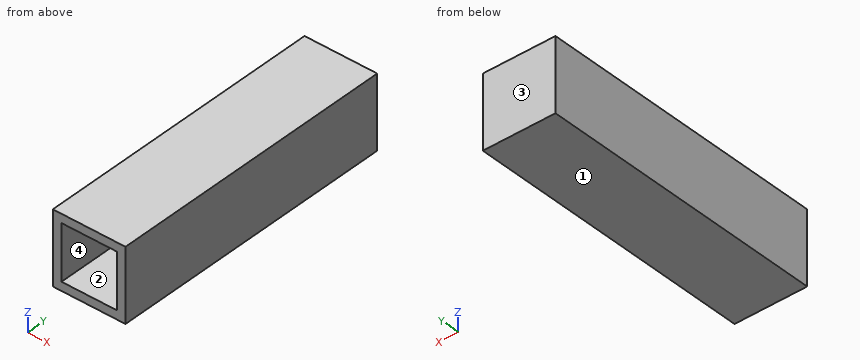
```python
from build123d import *

# Parameters (mm, degrees)
SKETCH2_W             = 25
SKETCH2_H             = 25
BOSS_EXTRUDE2_DEPTH   = 100
SHELL2_T              = -3
BODY_MOVE_COPY1_ANGLE = 180


with BuildPart() as part:
    # Sketch2 → Boss-Extrude2 (new body)
    with BuildSketch(Plane(origin=(0, 0, 0), x_dir=(1, 0, 0), z_dir=(0, 1, 0))):
        Rectangle(SKETCH2_W, SKETCH2_H)
    extrude(amount=BOSS_EXTRUDE2_DEPTH)

    # Shell2
    shell2_openings = [part.faces().sort_by_distance(p)[0] for p in [
        (0, 100, 0),
    ]]
    offset(amount=SHELL2_T, openings=shell2_openings, kind=Kind.INTERSECTION)


with BuildPart() as part_1:
    # Body-Move/Copy1: moved
    add(part.part.rotate(Axis((0, 50, 0), (0, 0, 1)), BODY_MOVE_COPY1_ANGLE))


solid = part_1.part
```
Read the model definition and answer for the solid it produces. Units are mm, in the model's axes. Face numbers are marked on the shaded views. Give positions to 0.01 mm unless a question says otherwise; leave off trailing zeros. Loops run counter-clockwise (first coordinate to the right, second up) from the corner with the lowest first, then second, coordinate; pieces in that order, holes last.
Item 1: This flat-tipped pin is pushed along its axis until it touches: pin 1 Ø1.5 at (x, z) = (-4.5, -1.5) entering from -Y. Where does it stop, or does it pass through?
Item 2: The part is cut by section C-C (z = -8). Write down the section's boundary in (x, y), and give its area (3 significant figures).
Item 3: The part is cut by section B-B (x = -4.5). Write down the section's boundary in (y, z), and give its area (3 significant figures).
Item 4: Find the intervals of material crossed by line 1 along X through (y, z) = (15, 6.75); line 2 along Y through (x, z) = (0.25, -5.5), in increasing order.
Item 5: The mould has two halves that part along Z. Classify the marked faces 1, 2, 3 and 4: released by +Z, released by -Z, zero draft, split by the parting line, or undercut.
Item 6: The part is cut by section A-A (y = 34). Write down the section's boundary in (x, z).
Taken from the geometry:
1. pin 1: stops at y = 97
2. outline: (-12.5, 0) - (-9.5, 0) - (-9.5, 97) - (9.5, 97) - (9.5, 0) - (12.5, 0) - (12.5, 100) - (-12.5, 100) - close
2. area: 657 mm2
3. outline: (0, -12.5) - (100, -12.5) - (100, 12.5) - (0, 12.5) - (0, 9.5) - (97, 9.5) - (97, -9.5) - (0, -9.5) - close
3. area: 657 mm2
4. line 1: x = -12.5 to -9.5, 9.5 to 12.5
4. line 2: y = 97 to 100
5. face 1: released by -Z
5. face 2: undercut
5. face 3: zero draft
5. face 4: undercut
6. outline: (-12.5, -12.5) - (12.5, -12.5) - (12.5, 12.5) - (-12.5, 12.5) - close; hole (-9.5, -9.5) - (9.5, -9.5) - (9.5, 9.5) - (-9.5, 9.5) - close
